Check sheet for the modelled part. Datum: model origin and axes. Units: mm. A direction names the side the tool comes from. Coordinates: 2 decimals unless noted, no trailing zeros. Write each loop counter-clockwise with the first axis right and the second up, starting at its lowest first coordinate (ties: lowest second). Pieces come first, ordered by that corner, then holes. Notation, with made-up numbers: (75, -32) -> (82, -32) arc R26 ccw to (82, -11) -> close; hole circle Ø2 at (77.5, 29.25). An arc over 180 degrees is marked (long way). One line per item, written item: value. Start each with the question number.
1) Scan lines: line 1 along Z through (x, y) = (-32.5, -6); line 2 along Z through (x, y) = (-79.5, 12.75); line 3 along Y through (x, z) = (-57, 12.5). Record each from-to range of solid material in increasing order. Write a range as [from, to].
2) Sectioned sample at B-B on z = 21.5. Enter the section's corners in (x, y).
3) Gauge pin test, flat ends, axial feed: P1, Ø1.9, axis at x = 0, y = 6.79, coming from the -Z side; P2, Ø5, axis at x = -32.96, z = 17.11, coming from the +Y side. Record the tip position at first contact, or that the pin passes through.
4) Sectioned sample at A-A on x = 82. Enter the section's corners in (y, z).
5) Set-up check for faces 1 (the flat face through (-128.21, -6, 7)), 2 (the flat face through (-3, 6, 2.54)): record each of +Z, -Z, +X, -X, +Y, -Y from which the full face is reachable in a straight line by a thin tool's end or side.
```python
from build123d import *

# Parameters (mm, degrees)
F0_W     = 254
F0_H     = 25.4
F1_DEPTH = 25.4
F2_T     = -2.54
F4_D     = 3.175
F6_D     = 3.175


with BuildPart() as f1:
    # F0 (on Top) → F1 (new body)
    with BuildSketch(Plane.XY):
        with Locations((-1.209586, 4.511842)):
            Rectangle(F0_W, F0_H)
    extrude(amount=F1_DEPTH)

    # F2
    f2_openings = [f1.faces().sort_by_distance(p)[0] for p in [
        (-1.209586, 4.511842, 25.4),
        (-1.209586, 17.211842, 12.7),
        (125.790414, 4.511842, 12.7),
        (-128.209586, 4.511842, 12.7),
    ]]
    offset(amount=F2_T, openings=f2_openings)

    # F4 (through all)
    with Locations(Plane.XY.offset(2.54)):
        with Locations((63.5, 6.789771), (0, 6.789771), (-64.709586, 6.789771)):
            Hole(F4_D / 2)

    # F6 (through all)
    with Locations(Plane(origin=(0, -5.648158, 0), x_dir=(-1, 0, 0), z_dir=(0, 1, 0))):
        with Locations((-43.240414, 8.641747), (-43.240414, 17.108414), (32.959586, 17.108414), (32.959586, 8.641747)):
            Hole(F6_D / 2)


solid = f1.part
```
Answers:
1. line 1: z = [0, 7.12], [10.16, 15.59], [18.63, 25.4]
1. line 2: z = [0, 2.54]
1. line 3: y = [-8.19, -5.65]
2. outline: (-128.21, -8.19) -> (125.79, -8.19) -> (125.79, -5.65) -> (-128.21, -5.65) -> close
3. P1: passes through
3. P2: stops at y = -5.65
4. outline: (-8.19, 0) -> (17.21, 0) -> (17.21, 2.54) -> (-5.65, 2.54) -> (-5.65, 25.4) -> (-8.19, 25.4) -> close
5. face 1: +Z, -Z, -X, +Y, -Y
5. face 2: +Z, +X, -X, +Y
